Verification items for the finished model (mm, model axes). A direction names the side the tool comes from. Coordinates: 2 decimals unless noted, no trailing zeros. Write each loop counter-clockwise with the first axis right and the second up, starting at its lowest first coordinate (ties: lowest second). Pieces come first, ordered by that corner, then holes. Notation, with made-up numbers: (8.25, -24) - (47.25, -24) arc R15 ccw to (47.25, -11) - close; hole circle Ø6 at (-10.5, 67). An arc over 180 degrees is marked (long way). Answer as CSV lines item,"result". Start each with the question number.
```python
from build123d import *

# Parameters (mm, degrees)
EXTRUDE1_DEPTH     = 2.5
CUT_EXTRUDE1_REACH = 7.75
SKETCH2_R          = 0.885
SKETCH2_W          = 4.04
SKETCH2_H          = 0.3
SKETCH2_W_2        = 0.84
SKETCH2_W_3        = 2.115


with BuildPart() as part:
    # Sketch1 → Extrude1 (new body)
    with BuildSketch(Plane.XY):
        Polygon((-1.6, 1), (1.6, 1), (1.6, 0), (6.325, 0), (6.325, 5.75), (1.6, 5.75), (1.6, 4.75), (-1.6, 4.75), (-1.6, 5.75), (-6.325, 5.75), (-6.325, 0), (-1.6, 0), align=None)
    extrude(amount=EXTRUDE1_DEPTH)

    # Sketch2 → Cut-Extrude1 (cut, up to next)
    with BuildSketch(Plane(origin=(0, 5.75, 0), x_dir=(-1, 0, 0), z_dir=(0, 1, 0)), mode=Mode.PRIVATE) as cut_extrude1_sk1:
        with Locations((3.325, 1.3)):
            Circle(SKETCH2_R)
    cut_extrude1_tool1 = extrude(cut_extrude1_sk1.sketch, amount=-CUT_EXTRUDE1_REACH, mode=Mode.PRIVATE) & part.part
    add(cut_extrude1_tool1.solids().sort_by_distance((-3.325, 5.75, 1.3))[0], mode=Mode.SUBTRACT)
    # Sketch2 → Cut-Extrude1 (cut, up to next)
    with BuildSketch(Plane(origin=(0, 5.75, 0), x_dir=(-1, 0, 0), z_dir=(0, 1, 0)), mode=Mode.PRIVATE) as cut_extrude1_sk2:
        with Locations((-3.325, 1.3)):
            Circle(SKETCH2_R)
    cut_extrude1_tool2 = extrude(cut_extrude1_sk2.sketch, amount=-CUT_EXTRUDE1_REACH, mode=Mode.PRIVATE) & part.part
    add(cut_extrude1_tool2.solids().sort_by_distance((3.325, 5.75, 1.3))[0], mode=Mode.SUBTRACT)
    # Sketch2 → Cut-Extrude1 (cut, up to next)
    with BuildSketch(Plane(origin=(0, 5.75, 0), x_dir=(-1, 0, 0), z_dir=(0, 1, 0)), mode=Mode.PRIVATE) as cut_extrude1_sk3:
        with Locations((-0.42, 2.35)):
            Rectangle(SKETCH2_W, SKETCH2_H)
    cut_extrude1_tool3 = extrude(cut_extrude1_sk3.sketch, amount=-CUT_EXTRUDE1_REACH, mode=Mode.PRIVATE) & part.part
    add(cut_extrude1_tool3.solids().sort_by_distance((0.42, 5.75, 2.35))[0], mode=Mode.SUBTRACT)
    # Sketch2 → Cut-Extrude1 (cut, up to next)
    with BuildSketch(Plane(origin=(0, 5.75, 0), x_dir=(-1, 0, 0), z_dir=(0, 1, 0)), mode=Mode.PRIVATE) as cut_extrude1_sk4:
        with Locations((2.02, 2.35)):
            Rectangle(SKETCH2_W_2, SKETCH2_H)
    cut_extrude1_tool4 = extrude(cut_extrude1_sk4.sketch, amount=-CUT_EXTRUDE1_REACH, mode=Mode.PRIVATE) & part.part
    add(cut_extrude1_tool4.solids().sort_by_distance((-2.02, 5.75, 2.35))[0], mode=Mode.SUBTRACT)
    # Sketch2 → Cut-Extrude1 (cut, up to next)
    with BuildSketch(Plane(origin=(0, 5.75, 0), x_dir=(-1, 0, 0), z_dir=(0, 1, 0)), mode=Mode.PRIVATE) as cut_extrude1_sk5:
        with Locations((-5.2675, 2.35)):
            Rectangle(SKETCH2_W_3, SKETCH2_H)
    cut_extrude1_tool5 = extrude(cut_extrude1_sk5.sketch, amount=-CUT_EXTRUDE1_REACH, mode=Mode.PRIVATE) & part.part
    add(cut_extrude1_tool5.solids().sort_by_distance((5.2675, 5.75, 2.35))[0], mode=Mode.SUBTRACT)
    # Sketch2 → Cut-Extrude1 (cut, up to next)
    with BuildSketch(Plane(origin=(0, 5.75, 0), x_dir=(-1, 0, 0), z_dir=(0, 1, 0)), mode=Mode.PRIVATE) as cut_extrude1_sk6:
        with Locations((5.2675, 2.35)):
            Rectangle(SKETCH2_W_3, SKETCH2_H)
    cut_extrude1_tool6 = extrude(cut_extrude1_sk6.sketch, amount=-CUT_EXTRUDE1_REACH, mode=Mode.PRIVATE) & part.part
    add(cut_extrude1_tool6.solids().sort_by_distance((-5.2675, 5.75, 2.35))[0], mode=Mode.SUBTRACT)


solid = part.part
```
1. Cross-section at C-C (x = 3). Record the cut outline in (y, z), and give its area (3 significant figures).
2. Draft check along X on faces 4 (the face through (6.325, 3, 1)), 5 (the face through (4.5, 0, 1.2)), 6 (the face through (1.6, 5, 1)). Enter one of: pulls with the +X half, pulls with the -X half, needs draft (parallel to the pull), parting line crosses it, or undercut.
3. Cross-section at B-B (y = 3.3). Record the cut outline in (x, z) (3 decimals), and give its area (3 significant figures).
4. Cross-section at D-D (z = 0.55). Record the cut outline in (x, y) (3 decimals).
5. Access from +Z, -Z, +X, -X, +Y, -Y to the whole of each face (thin tool, end or side, straight path). Record for faces 1 (the face through (1.6, 0.5, 1.1)), 2 (the face through (5, 3, 2.2)), 3 (the face through (-5, 3, 2.2)).
6. Scan lines: line 1 along X through (y, z) = (1.1, 1.4) (3 decimals); line 2 along X through (y, z) = (3.7, 0.65) (3 decimals); line 3 along X through (y, z) = (5.15, 0.7) (3 decimals). Record each from-to range of solid material in increasing order. Write a range as from..to.
7. Cross-section at A-A (z = 1.3). Record the cut outline in (x, y) (3 decimals).
8. Depth check by flat-ended pin: P1, Ø1, axis at x = -1, z = 1, coming from the +Y side. Enter the tip coordinate at first touch or a pass-through.
Completed:
1,outline,"(0, 0) - (5.75, 0) - (5.75, 0.48) - (0, 0.48) - close; (0, 2.12) - (5.75, 2.12) - (5.75, 2.5) - (0, 2.5) - close"
1,area,"4.91 mm2"
2,face 4,"pulls with the +X half"
2,face 5,"needs draft"
2,face 6,"undercut"
3,outline,"(-6.325, 0) - (6.325, 0) - (6.325, 2.2) - (4.21, 2.2) - (4.21, 2.5) - (2.44, 2.5) - (2.44, 2.2) - (-2.44, 2.2) - (-2.44, 2.5) - (-4.21, 2.5) - (-4.21, 2.2) - (-6.325, 2.2) - close; hole circle Ø1.77 at (-3.325, 1.3); hole circle Ø1.77 at (3.325, 1.3)"
3,area,"24.0 mm2"
4,outline,"(-6.325, 0) - (-3.795, 0) - (-3.795, 5.75) - (-6.325, 5.75) - close; (-2.855, 0) - (-1.6, 0) - (-1.6, 1) - (1.6, 1) - (1.6, 0) - (2.855, 0) - (2.855, 5.75) - (1.6, 5.75) - (1.6, 4.75) - (-1.6, 4.75) - (-1.6, 5.75) - (-2.855, 5.75) - close; (3.795, 0) - (6.325, 0) - (6.325, 5.75) - (3.795, 5.75) - close"
5,face 1,"+Z, -Z, -Y"
5,face 2,"+Z, +X, +Y, -Y"
5,face 3,"+Z, -X, +Y, -Y"
6,line 1,"x = -6.325..-4.204, -2.446..2.446, 4.204..6.325"
6,line 2,"x = -6.325..-3.926, -2.724..2.724, 3.926..6.325"
6,line 3,"x = -6.325..-3.976, -2.674..-1.6, 1.6..2.674, 3.976..6.325"
7,outline,"(-6.325, 0) - (-4.21, 0) - (-4.21, 5.75) - (-6.325, 5.75) - close; (-2.44, 0) - (-1.6, 0) - (-1.6, 1) - (1.6, 1) - (1.6, 0) - (2.44, 0) - (2.44, 5.75) - (1.6, 5.75) - (1.6, 4.75) - (-1.6, 4.75) - (-1.6, 5.75) - (-2.44, 5.75) - close; (4.21, 0) - (6.325, 0) - (6.325, 5.75) - (4.21, 5.75) - close"
8,P1,"stops at y = 4.75"
